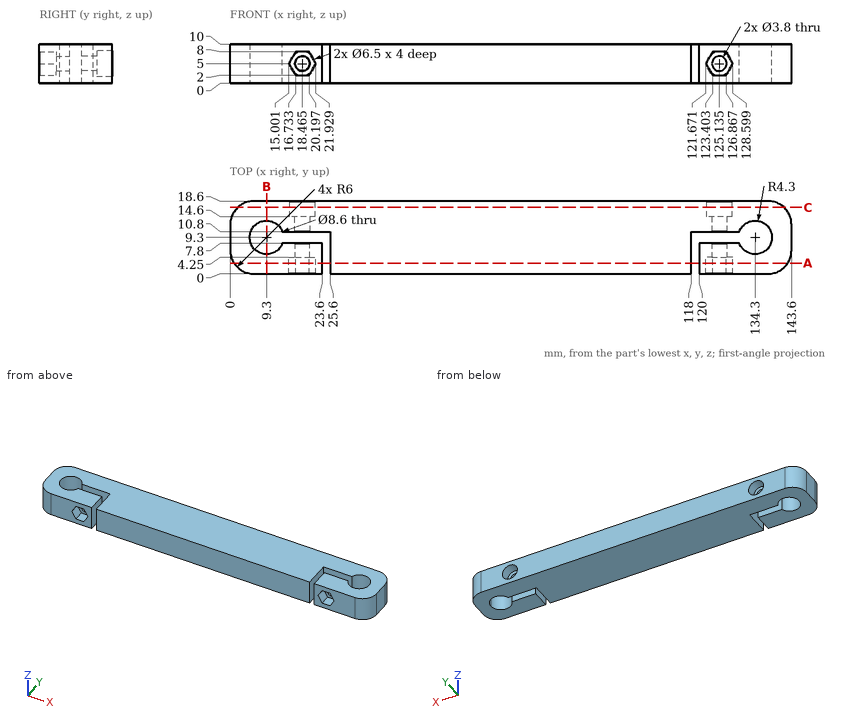
Geometry: see drawing. Coordinates: mm, zero at the bounding-box minimum. Coordinates: 2 decimals unless noted, no trailing zeros. Order: outer loops, then holes, each group sorted by start corner. A loop starts at its lowest first (then second) coordinate and runs counter-clockwise, first axis right, second up. Notation, with made-up numbers: M 39.5,11.25 L 55.5,11.25 A21 ccw 55.5,41.25 Z; hole C 24.5,-7 d8. An arc over 180 degrees is marked long. Write item = value, one per line. Start each with the question number.
(1) First-contact query: P1, Ø1.5, axis at y = 16, z = 7.5, coming from the +X side; P2, Ø2.5, axis at y = 3.5, z = 7.5, coming from the -X side; P3, Ø1, axis at y = 4, z = 8.5, coming from the +X side. Flat tips, straight axial feed; report the tip coordinate or a pass-through.
(2) Section A-A on y = 2.75. Output: boundary loops of the cut face in (x, z), and give its area (3 significant figures).
(3) Line query: line 1 along X through (y, z) = (9, 5.5); line 2 along X through (y, z) = (16.55, 5) (1 decimal); line 3 along X through (y, z) = (12.25, 3.5). Output: solid intervals per line, ascending. Write a range as [from, to].
(4) Section C-C on y = 17. Give the number of separate pieces and of enclosed holes in the cut face, and give its area (3 significant figures).
(5) Section B-B on x = 9.3. Output: boundary loops of the cut face in (y, z), and give its area (4 significant figures).
Result set:
q1.P1 = 142.98
q1.P2 = 0.13
q1.P3 = 143.41
q2.outline = M 0.96,0 L 23.6,0 L 23.6,10 L 0.96,10 Z; M 25.6,0 L 118,0 L 118,10 L 25.6,10 Z; M 120,0 L 142.64,0 L 142.64,10 L 120,10 Z; hole M 15,5 L 16.73,2 L 20.2,2 L 21.93,5 L 20.2,8 L 16.73,8 Z; hole M 121.67,5 L 123.4,2 L 126.87,2 L 128.6,5 L 126.87,8 L 123.4,8 Z
q2.area = 1,310 mm²
q3.line_1 = [0, 5.01], [25.6, 118], [138.59, 143.6]
q3.line_2 = [1.5, 15.2], [21.7, 121.9], [128.4, 142.1]
q3.line_3 = [0, 6.17], [12.43, 17.3], [19.63, 123.97], [126.3, 131.17], [137.43, 143.6]
q4.separate_pieces = 1
q4.enclosed_holes = 2
q4.area = 1,330 mm²
q5.outline = M 0,0 L 5,0 L 5,10 L 0,10 Z; M 13.6,0 L 18.6,0 L 18.6,10 L 13.6,10 Z
q5.area = 100.0 mm²
